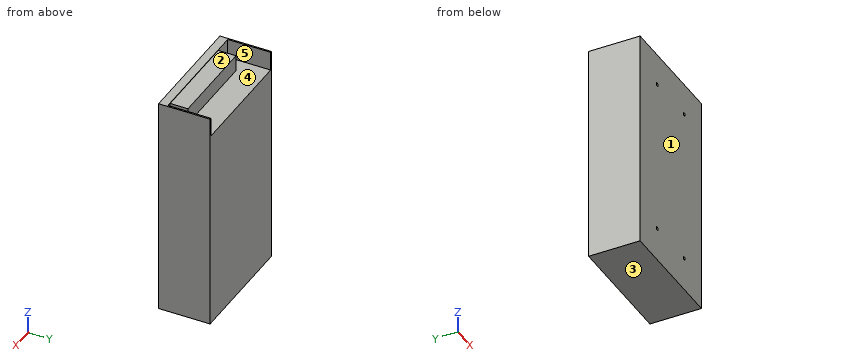
from build123d import *

# Parameters (mm, degrees)
SKETCH1_W           = 113.03
SKETCH1_H           = 213.36
BOSS_EXTRUDE1_DEPTH = 49.53
SKETCH2_W           = 110.0836
SKETCH2_H           = 18.415
CUT_EXTRUDE1_DEPTH  = 41.275
SKETCH3_W           = 88.4682
SKETCH3_H           = 15.494
BOSS_EXTRUDE2_DEPTH = 17.0942
SKETCH4_R           = 1.5875
CUT_EXTRUDE2_DEPTH  = 5


with BuildPart() as part:
    # Sketch1 → Boss-Extrude1 (new body)
    with BuildSketch(Plane(origin=(0, 0, 0), x_dir=(1, 0, 0), z_dir=(0, 1, 0))):
        with Locations((56.515, 106.68)):
            Rectangle(SKETCH1_W, SKETCH1_H)
    extrude(amount=BOSS_EXTRUDE1_DEPTH)

    # Sketch2 → Cut-Extrude1 (cut)
    with BuildSketch(Plane(origin=(0, 49.53, 0), x_dir=(1, 0, 0), z_dir=(0, 1, 0))):
        with Locations((56.515, 9.2075)):
            Rectangle(SKETCH2_W, SKETCH2_H)
    extrude(amount=-CUT_EXTRUDE1_DEPTH, mode=Mode.SUBTRACT)

    # Sketch3 → Boss-Extrude2 (add)
    with BuildSketch(Plane(origin=(0, 8.255, 0), x_dir=(1, 0, 0), z_dir=(0, 1, 0))):
        with Locations((63.1825, 8.255)):
            Rectangle(SKETCH3_W, SKETCH3_H)
    extrude(amount=BOSS_EXTRUDE2_DEPTH)

    # Sketch4 → Cut-Extrude2 (cut)
    with BuildSketch(Plane.XZ):
        with Locations(Location((81.515, -180.86, 0), (0, 0, 270))):
            Circle(SKETCH4_R)
        with Locations(Location((31.515, -180.86, 0), (0, 0, 270))):
            Circle(SKETCH4_R)
        with Locations(Location((81.515, -30.86, 0), (0, 0, 270))):
            Circle(SKETCH4_R)
        with Locations(Location((31.515, -30.86, 0), (0, 0, 270))):
            Circle(SKETCH4_R)
    extrude(amount=-CUT_EXTRUDE2_DEPTH, mode=Mode.SUBTRACT)


solid = part.part
CAD build for the part. Positions are in the model's coordinates, mm. Face numbers are marked on the shaded views. A direction names the side the tool comes from. Round coordinates to 2 decimals unless told otherwise and drop trailing zeros. Write each loop counter-clockwise with the first axis right and the second up, starting at its lowest first coordinate (ties: lowest second). Pieces come first, ordered by that corner, then holes.
(1) Slice it at A-A, the plane y = 20. Write the cut outline in (x, z) (3 decimals).
(2) Probe line 1 along X through (y, z) = (3.35, -30.86); line 2 along Z through (x, y) = (28, 11) (3 decimals); line 3 along Y through (x, z) = (57, -15). List the from-to ranges inside material, lowest first.
(3) Mould opens along Z. For the marked faces 3, 4 and 5 say: pulls with the +Z half, pulls with the -Z half, needs draft (parallel to the pull), parting line crosses it, or undercut.
(4) 3-axis set-ups, long thin cutter, end or side, ignore diameter. For the marked faces 1 and 2: which of +Z, -Z, +X, -X, +Y, -Y reach the whole face in a straight line?
(5) Drop flat-ended pins along their axis: P1, Ø1, axis at x = 81, z = -31.5, coming from the -Y side; P2, Ø12.5, axis at x = 42.5, y = 21, coming from the +Z side; P3, Ø9, axis at x = 39, z = -5, coming from the +Y side. Give the stop position or say it passes through.
(6) Slice it at B-B, the plane x = 77. Write the cut outline in (y, z) (3 decimals), and give its area (3 significant figures).
From the geometry:
1. outline: (0, -213.36) - (113.03, -213.36) - (113.03, 0) - (111.557, 0) - (111.557, -18.415) - (1.473, -18.415) - (1.473, 0) - (0, 0) - close; (18.948, -16.002) - (107.417, -16.002) - (107.417, -0.508) - (18.948, -0.508) - close
2. line 1: x = 0 to 29.93, 33.1 to 79.93, 83.1 to 113.03
2. line 2: z = -213.36 to -18.415, -16.002 to -0.508
2. line 3: y = 0 to 25.35
3. face 3: pulls with the -Z half
3. face 4: undercut
3. face 5: needs draft
4. face 1: +Z, -Z, +X, -X, -Y
4. face 2: +Z, +Y
5. P1: stops at y = 5
5. P2: stops at z = -0.51
5. P3: stops at y = 25.35
6. outline: (0, -213.36) - (49.53, -213.36) - (49.53, -18.415) - (8.255, -18.415) - (8.255, -16.002) - (25.349, -16.002) - (25.349, -0.508) - (8.255, -0.508) - (8.255, 0) - (0, 0) - close
6. area: 10,100 mm2
